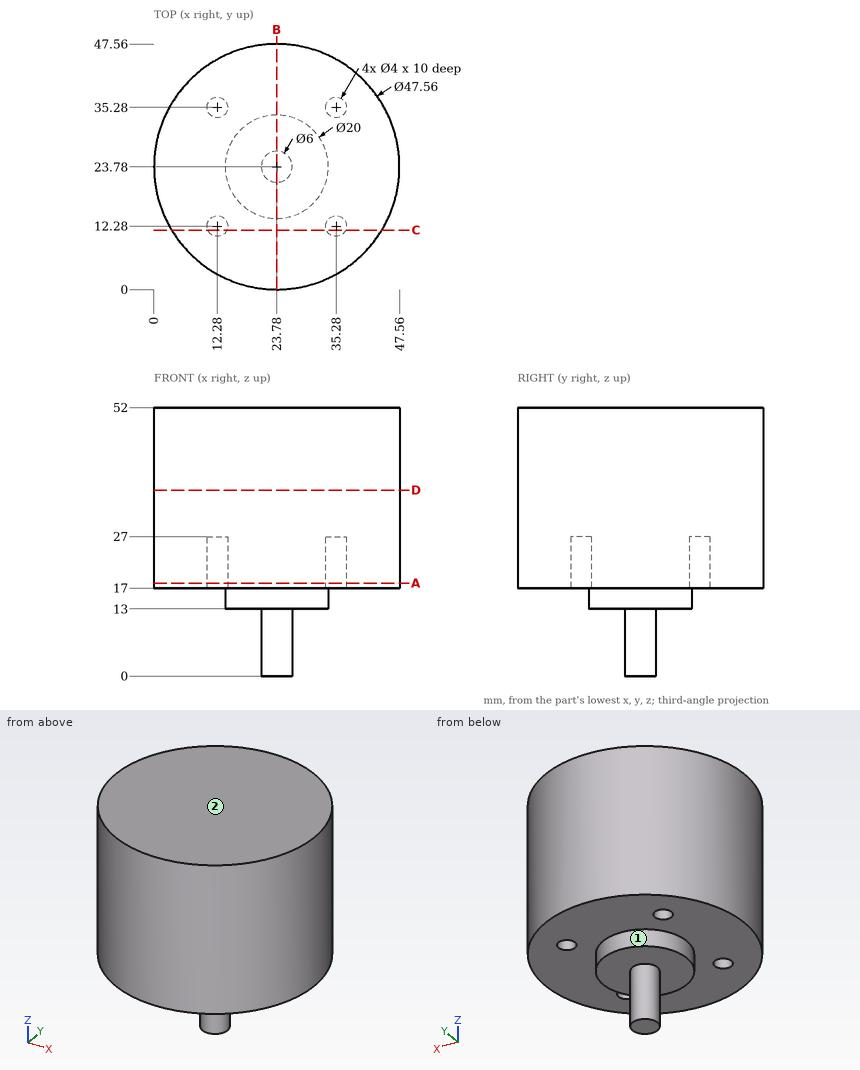
Check sheet for the drawn part. Datum: minimum x, y, z corner. Units: mm. A direction names the side the tool comes from. Give positions to 0.01 mm unless a question says otherwise; leave off trailing zeros. Order: outer loops, then holes, each group sorted by start corner. A loop starts at its lowest first (then second) coordinate and runs counter-clockwise, first axis right, second up. Notation, with made-up numbers: (55, -28) -> (61, -28) arc R19 cw to (61, -6) -> close; hole circle Ø3 at (-12.75, 14). An arc over 180 degrees is marked (long way). Use a Markdown table: item, result.
1) Depth check by flat-ended pin: pin 1 Ø4.5 at (x, y) = (13, 13) entering from -Z; pin 2 Ø4 at (y, z) = (37, 27) entering from +X; pin 3 Ø2.5 at (x, y) = (12.28, 12.28) entering from -Z. Enter the tip coordinate at first touch or a pass-through.
Results:
| item | result |
|---|---|
| pin 1 | z = 17 |
| pin 2 | x = 44.75 |
| pin 3 | z = 27 |
2) Material ranges on probe 1 along X at (y, z) = (12, 25); probe 2 along Y at (x, z) = (35.28, 23); probe 3 along Z at (x, y) = (7, 36.5), recorded low to high.
Results:
| item | result |
|---|---|
| probe 1 | 3.12 to 10.3, 14.26 to 33.3, 37.26 to 44.44 |
| probe 2 | 2.97 to 10.28, 14.28 to 33.28, 37.28 to 44.59 |
| probe 3 | 17 to 52 |
3) Tool access check on the marked faces 1 and 2. Record the directions out of +Z, -Z, +X, -X, +Y, -Y that give a thin tool (end or side, any length) a straight path to the whole face; none if there is none.
Results:
| item | result |
|---|---|
| face 1 | -Z |
| face 2 | +Z, +X, -X, +Y, -Y |
4) Section check C-C, the plane y = 11.5. Record the boundary of the cut face in (x, z), then the cut area to 3 significant figures.
Results:
| item | result |
|---|---|
| outline | (3.42, 17) -> (10.44, 17) -> (10.44, 27) -> (14.12, 27) -> (14.12, 17) -> (33.44, 17) -> (33.44, 27) -> (37.12, 27) -> (37.12, 17) -> (44.14, 17) -> (44.14, 52) -> (3.42, 52) -> close |
| area | 1,350 mm² |
5) Section check D-D, the plane z = 36. Record the boundary of the cut face in (x, y).
Results:
| item | result |
|---|---|
| outline | circle Ø47.56 at (23.78, 23.78) |
6) Section check A-A, the plane z = 18. Record the boundary of the cut face in (x, y).
Results:
| item | result |
|---|---|
| outline | circle Ø47.56 at (23.78, 23.78); hole circle Ø4 at (12.28, 12.28); hole circle Ø4 at (12.28, 35.28); hole circle Ø4 at (35.28, 12.28); hole circle Ø4 at (35.28, 35.28) |
7) Section check B-B, the plane x = 23.78. Record the boundary of the cut face in (y, z).
Results:
| item | result |
|---|---|
| outline | (0, 17) -> (13.78, 17) -> (13.78, 13) -> (20.78, 13) -> (20.78, 0) -> (26.78, 0) -> (26.78, 13) -> (33.78, 13) -> (33.78, 17) -> (47.56, 17) -> (47.56, 52) -> (0, 52) -> close |
